Design review of the part built by this model. Coordinates are the model's own, in mm. Give positions to 0.01 mm unless a question says otherwise; leave off trailing zeros. Loops run counter-clockwise (first coordinate to the right, second up) from the corner with the lowest first, then second, coordinate; pieces in that order, holes last. Notation, with made-up numbers: (64, 50.5) -> (79, 50.5) arc R22 cw to (79, 57.5) -> close; hole circle Ø7 at (17.25, 14.25). An arc over 180 degrees is marked (long way). Answer as CSV lines item,"result".
from build123d import *

# Parameters (mm, degrees)
F0_W         = 142.9656147957
F0_H         = 80.8112323284
F1_DEPTH     = 3
F2_W         = 137.4550536275
F2_H         = 8.9848991483
F2_W_2       = 60.0944850594
F2_H_2       = 18.4983238578
F3_DEPTH     = 52.3
F4_W         = 39.2408655025
F4_H         = 21.6958951205
F5_DEPTH     = 25
F6_W         = 3.3521875739
F6_H         = 44.7733802721
F6_W_2       = 40.9712046385
F7_DEPTH     = 25
F8_W         = 102.604271844
F8_H         = 18.422623165
F9_DEPTH     = 25
F10_T1_DEPTH = 3
F10_T3_DEPTH = 60.941125497
F12_DEPTH    = 25
F14_DEPTH    = 25
F16_DEPTH    = 25
F17_W        = 93.9226467162
F17_H        = 5.0384774804
F18_DEPTH    = 1.4789979905
F19_W        = 52.2845312953
F19_H        = 2.1970570087
F20_DEPTH    = 0.8268505335
F21_DEPTH    = 0.7327459753
F22_W        = 3.9923638105
F22_H        = 1.5595965087
F23_DEPTH    = 65.8853985369
F24_W        = 7.4088871479
F24_H        = 1.9754432142
F25_DEPTH    = 1.11994287


# Not quite as in the source:
# - a fillet or chamfer that OpenCascade refuses, or shapes differently, is made with other operations: its cross-section is extruded or revolved along the edge and cut away or added


with BuildPart() as f1:
    # F0 (on Top) → F1 (new body)
    with BuildSketch(Plane.XY):
        Rectangle(F0_W, F0_H)
    extrude(amount=F1_DEPTH)

    # F2 (on face) → F3 (cut)
    with BuildSketch(Plane.XY.offset(3)):
        with Locations((2.7552805841, 33.0591509119)):
            Rectangle(F2_W, F2_H)
        with Locations((41.4355648682, 14.2965670675)):
            Rectangle(F2_W_2, F2_H_2)
    extrude(amount=-F3_DEPTH, mode=Mode.SUBTRACT)

    # F4 (on face) → F5 (cut)
    with BuildSketch(Plane.XY.offset(3)):
        with Locations((-13.8379565906, 10.8479475603)):
            Rectangle(F4_W, F4_H)
    extrude(amount=-F5_DEPTH, mode=Mode.SUBTRACT)

    # F6 (on face) → F7 (cut)
    with BuildSketch(Plane.XY.offset(3)):
        Polygon((98.6725464463, 0), (13.7504395097, 0), (13.7504395097, -5.2010240033), (17.1026270837, -5.2010240033), (17.1026270837, -49.9744042754), (13.7504395097, -49.9744042754), (13.7504395097, -55.2418604493), (98.6725464463, -55.2418604493), align=None)
        with Locations((15.4265332967, -27.5877141394)):
            Rectangle(F6_W, F6_H)
        with Locations((-6.7351628095, -27.5877141394)):
            Rectangle(F6_W_2, F6_H)
    extrude(amount=-F7_DEPTH, mode=Mode.SUBTRACT)

    # F8 (on face) → F9 (cut)
    with BuildSketch(Plane.XY.offset(3)):
        with Locations((62.6904582605, -4.1639064439)):
            Rectangle(F8_W, F8_H)
    extrude(amount=-F9_DEPTH, mode=Mode.SUBTRACT)

    # F10: fillet of radius 11.5882250994 on 7 edges, made by hand

    # F10_s2 → F10_t1 (join)
    with BuildSketch(Plane.XY):
        with BuildLine():
            ThreePointArc((22.9765474379, 23.5457289964), (14.7824348882, 20.1516164467), (11.3883223385, 11.957503897))
            Line((11.3883223385, 11.957503897), (11.3883223385, 23.5457289964))
            Line((11.3883223385, 23.5457289964), (22.9765474379, 23.5457289964))
        make_face()
        with BuildLine():
            ThreePointArc((-15.6325400293, -5.2010240033), (-23.826652579, -8.595136553), (-27.2207651287, -16.7892491027))
            Line((-27.2207651287, -16.7892491027), (-27.2207651287, -5.2010240033))
            Line((-27.2207651287, -5.2010240033), (-15.6325400293, -5.2010240033))
        make_face()
        with BuildLine():
            ThreePointArc((-33.4583893418, 10.1076700211), (-30.0642767921, 18.3017825708), (-21.8701642424, 21.6958951205))
            Line((-21.8701642424, 21.6958951205), (-33.4583893418, 21.6958951205))
            Line((-33.4583893418, 21.6958951205), (-33.4583893418, 10.1076700211))
        make_face()
        with BuildLine():
            ThreePointArc((-5.8057489387, 0), (2.388363611, 3.3941125497), (5.7824761607, 11.5882250994))
            Line((5.7824761607, 11.5882250994), (5.7824761607, 0))
            Line((5.7824761607, 0), (-5.8057489387, 0))
        make_face()
        with BuildLine():
            ThreePointArc((-33.4583893418, 11.5882250994), (-30.0642767921, 3.3941125497), (-21.8701642424, 0))
            Line((-21.8701642424, 0), (-33.4583893418, 0))
            Line((-33.4583893418, 0), (-33.4583893418, 11.5882250994))
        make_face()
        with BuildLine():
            ThreePointArc((5.7824761607, 10.1076700211), (2.388363611, 18.3017825708), (-5.8057489387, 21.6958951205))
            Line((-5.8057489387, 21.6958951205), (5.7824761607, 21.6958951205))
            Line((5.7824761607, 21.6958951205), (5.7824761607, 10.1076700211))
        make_face()
    extrude(amount=F10_T1_DEPTH)

    # F10_s4 → F10_t3 (cut)
    with BuildSketch(Plane.XY.offset(-28.9705627485)):
        with BuildLine():
            ThreePointArc((-0.1999027609, -5.2010240033), (7.9942097888, -1.8069114536), (11.3883223385, 6.3872010961))
            Line((11.3883223385, 6.3872010961), (11.3883223385, -5.2010240033))
            Line((11.3883223385, -5.2010240033), (-0.1999027609, -5.2010240033))
        make_face()
    extrude(amount=F10_T3_DEPTH, mode=Mode.SUBTRACT)

    # F11 (on face) → F12 (cut)
    with BuildSketch(Plane.XY.offset(3)):
        with BuildLine():
            Line((-71.4828073978, 25.5012605339), (-71.4828073978, -17.3091441393))
            ThreePointArc((-71.4828073978, -17.3091441393), (-66.7668008007, 4.0960581973), (-71.4828073978, 25.5012605339))
        make_face()
    extrude(amount=-F12_DEPTH, mode=Mode.SUBTRACT)

    # F13 (on face) → F14 (cut)
    with BuildSketch(Plane.XY.offset(3)):
        with BuildLine():
            ThreePointArc((-21.3245461018, -6.6952891353), (-30.1185964093, -13.4662376926), (-27.2207651287, -24.1799503565))
            Line((-27.2207651287, -24.1799503565), (-27.2207651287, -16.7892491027))
            ThreePointArc((-27.2207651287, -16.7892491027), (-25.6387183355, -10.944306275), (-21.3245461018, -6.6952891353))
        make_face()
        with BuildLine():
            ThreePointArc((-27.2207651287, -32.8327932205), (-29.4171017882, -37.101902666), (-32.9005867243, -40.4056161642))
            Line((-32.9005867243, -40.4056161642), (-27.2207651287, -40.4056161642))
            Line((-27.2207651287, -40.4056161642), (-27.2207651287, -32.8327932205))
        make_face()
        with BuildLine():
            ThreePointArc((-56.574376872, -40.4056161642), (-65.5880780241, -36.6447482344), (-71.4828073978, -28.8573801517))
            Line((-71.4828073978, -28.8573801517), (-71.4828073978, -40.4056161642))
            Line((-71.4828073978, -40.4056161642), (-56.574376872, -40.4056161642))
        make_face()
    extrude(amount=-F14_DEPTH, mode=Mode.SUBTRACT)

    # F15 (on face) → F16 (cut)
    with BuildSketch(Plane.XY.offset(3)):
        with BuildLine():
            Line((-32.9005867243, -5.2010240033), (-32.9005867243, -40.4056161642))
            ThreePointArc((-32.9005867243, -40.4056161642), (-29.4171017882, -37.101902666), (-27.2207651287, -32.8327932205))
            Line((-27.2207651287, -32.8327932205), (-27.2207651287, -24.1799503565))
            ThreePointArc((-27.2207651287, -24.1799503565), (-30.1185964093, -13.4662376926), (-21.3245461018, -6.6952891353))
            ThreePointArc((-21.3245461018, -6.6952891353), (-18.5749778542, -5.5808138595), (-15.6325400293, -5.2010240033))
            Line((-15.6325400293, -5.2010240033), (-32.9005867243, -5.2010240033))
        make_face()
    extrude(amount=-F16_DEPTH, mode=Mode.SUBTRACT)

    # F17 (on face) → F18 (join)
    with BuildSketch(Plane(origin=(0, 0, 0), x_dir=(1, 0, 0), z_dir=(0, 0, -1))):
        with Locations((-24.5214840397, -37.886377424)):
            Rectangle(F17_W, F17_H)
    extrude(amount=F18_DEPTH)

    # F19 (on face) → F20 (join)
    with BuildSketch(Plane(origin=(0, 0, 0), x_dir=(1, 0, 0), z_dir=(0, 0, -1))):
        with Locations((-39.829980582, -29.6652298421)):
            Rectangle(F19_W, F19_H)
        Polygon((-71.4828073978, -30.7637583464), (-65.9722462296, -30.7637583464), (-65.9722462296, -28.5667013377), (-13.6877149343, -28.5667013377), (-13.6877149343, -25.5012605339), (-71.4828073978, -25.5012605339), align=None)
    extrude(amount=F20_DEPTH)

    # F21 (add): a face of the model
    f21_faces = [f1.faces().sort_by_distance(p)[0] for p in [
        (-42.5852611661, 28.1325094402, -0.8268505335),
    ]]
    extrude(f21_faces, amount=F21_DEPTH)

    # F22 (on face) → F23 (join)
    with BuildSketch(Plane.XZ.offset(-25.5012605339)):
        with Locations((-38.7431830168, -0.7797982544)):
            Rectangle(F22_W, F22_H)
    extrude(amount=F23_DEPTH)

    # F24 (on face) → F25 (join)
    with BuildSketch(Plane(origin=(0, 0, -1.5595965087), x_dir=(1, 0, 0), z_dir=(0, 0, -1))):
        with Locations((-17.3921585083, -30.787916854)):
            Rectangle(F24_W, F24_H)
    extrude(amount=F25_DEPTH)


solid = f1.part
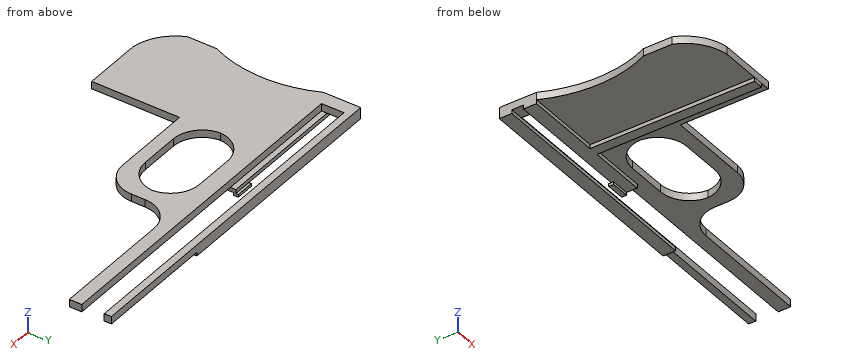
Q1. We need section B-B, the plane z = 2.1. State the section outline as (x, y) points.
Filled sheet:
outline,"(-71.48, -28.86) arc R18.73 ccw to (-56.57, -40.41) -> (-32.9, -40.41) -> (-32.9, -5.2) -> (-0.2, -5.2) arc R11.59 ccw to (11.39, 6.39) -> (11.39, 11.96) arc R11.59 cw to (22.98, 23.55) -> (71.48, 23.55) -> (71.48, 28.57) -> (-65.97, 28.57) -> (-65.97, 37.55) -> (71.48, 37.55) -> (71.48, 40.41) -> (-71.48, 40.41) -> (-71.48, 25.5) arc R50.94 cw to (-71.48, -17.31) -> close; hole (-33.43, 10.85) arc R11.59 ccw to (-21.87, 0) -> (-5.81, 0) arc R11.59 ccw to (5.76, 10.85) arc R11.59 ccw to (-5.81, 21.7) -> (-21.87, 21.7) arc R11.59 ccw to start"
Q2. To check wall thickness, follow probe 1 along Y at (x, z) = (32.5, 0.75); probe 2 along Y at (x, z) = (4, -0.05); probe 3 along X at (y, z) = (11, -0.95). State the ranges of each line that lie inside material, in increasing order. Write a range as from..to.
Filled sheet:
probe 1,"y = 23.55..28.57, 37.55..40.41"
probe 2,"y = 35.37..40.41"
probe 3,"x = -40.74..-36.75"
Q3. We need section D-D, the plane y = -27. State the section outline as (x, z) points.
Filled sheet:
outline,"(-71.48, 0) -> (-40.74, 0) -> (-40.74, -1.56) -> (-36.75, -1.56) -> (-36.75, 0) -> (-32.9, 0) -> (-32.9, 3) -> (-71.48, 3) -> close"
Q4. We need section C-C, the plane x = -27.5. State the section outline as (y, z) points.
Filled sheet:
outline,"(-5.2, 0) -> (1.46, 0) -> (1.46, 3) -> (-5.2, 3) -> close; (20.24, 0) -> (25.5, 0) -> (25.5, -1.56) -> (30.76, -1.56) -> (30.76, 0) -> (28.57, 0) -> (28.57, 3) -> (20.24, 3) -> close; (35.37, -1.48) -> (40.41, -1.48) -> (40.41, 3) -> (37.55, 3) -> (37.55, 0) -> (35.37, 0) -> close"
Q5. We need section A-A, the plane x = 31. State the section outline as (y, z) points.
Filled sheet:
outline,"(23.55, 0) -> (28.57, 0) -> (28.57, 3) -> (23.55, 3) -> close; (37.55, 0) -> (40.41, 0) -> (40.41, 3) -> (37.55, 3) -> close"
Q6. Clearance check with flat-ended pins moving along their axes: pin 1 Ø1.2 at (x, z) = (-18, -2.5) entering from +Y; pin 2 Ø0.5 at (x, y) = (-19, 31.5) entering from +Z; pin 3 Ø1.5 at (x, z) = (46.5, 1) entering from -Y. State where each tip first meets the part, or that it passes through.
Filled sheet:
pin 1,"stops at y = 31.78"
pin 2,"stops at z = -1.56"
pin 3,"stops at y = 23.55"
